Could you check a few things on this drawing? It's one solid part, dimensions in mm from its lowest x, y, z. Coordinates: 2 decimals unless noted, no trailing zeros. Order: outer loops, then holes, each group sorted by start corner. A loop starts at its lowest first (then second) coordinate and runs counter-clockwise, first axis right, second up. Notation, with made-up numbers: M 13,89.25 L 43,89.25 A19 ccw 43,114.25 Z; hole C 9.5,52 d3. An arc over 180 degrees is marked long. Write item = value, one per line. Start each with the question number.
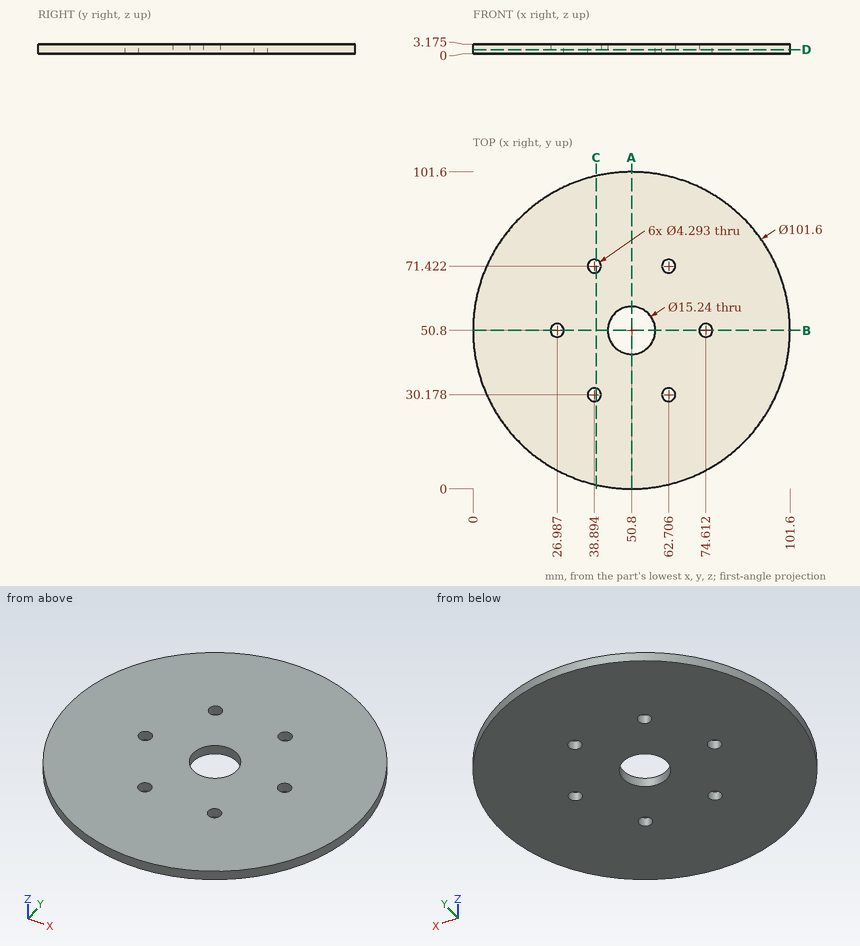
(1) Imagine slicing it at D-D on z = 1.35. List the corners of the cut face in (x, y) for me, plus the area to 3 significant figures.
(2) Imagine slicing it at C-C on x = 39.5. List the corners of the cut face in (y, z) for me (1 decimal).
(3) Imagine slicing it at B-B on y = 50.8. List the corners of the cut face in (x, z) for me (1 decimal).
(4) Will this pin go through, and if not, where does the flat tip stop? P1, Ø2.5, axis at x = 38.89, y = 30.18, coming from the -Z side.
(5) Imagine slicing it at A-A on x = 50.8. List the corners of the cut face in (y, z) for me (1 decimal).
(6) Please list where these lines run through material, in increasing order: probe 1 along Y at (x, z) = (50.8, 1.85); probe 2 along X at (y, z) = (70, 3) (1 decimal); probe 3 along Y at (x, z) = (48.5, 0.45) (1 decimal). Write a range as from..to.
Response:
q1.outline = C 50.8,50.8 d101.6; hole C 26.99,50.8 d4.29; hole C 38.89,30.18 d4.29; hole C 38.89,71.42 d4.29; hole C 50.8,50.8 d15.24; hole C 62.71,30.18 d4.29; hole C 62.71,71.42 d4.29; hole C 74.61,50.8 d4.29
q1.area = 7,840 mm2
q2.outline = M 1.3,0 L 28.1,0 L 28.1,3.2 L 1.3,3.2 Z; M 32.2,0 L 69.4,0 L 69.4,3.2 L 32.2,3.2 Z; M 73.5,0 L 100.3,0 L 100.3,3.2 L 73.5,3.2 Z
q3.outline = M 0,0 L 24.8,0 L 24.8,3.2 L 0,3.2 Z; M 29.1,0 L 43.2,0 L 43.2,3.2 L 29.1,3.2 Z; M 58.4,0 L 72.5,0 L 72.5,3.2 L 58.4,3.2 Z; M 76.8,0 L 101.6,0 L 101.6,3.2 L 76.8,3.2 Z
q4.P1 = through
q5.outline = M 0,0 L 43.2,0 L 43.2,3.2 L 0,3.2 Z; M 58.4,0 L 101.6,0 L 101.6,3.2 L 58.4,3.2 Z
q6.probe_1 = 0..43.18, 58.42..101.6
q6.probe_2 = 3.8..37.3, 40.5..61.1, 64.3..97.8
q6.probe_3 = 0.1..43.5, 58.1..101.5
